```python
from build123d import *

# Parameters (mm, degrees)
BOSS_EXTRUDE1_DEPTH            = 3
SKETCH2_R                      = 3.5
BOSS_EXTRUDE2_DEPTH            = 1.5
M3_CLEARANCE_HOLE1_D           = 3.6
M3_CLEARANCE_HOLE1_ON_FACE_2_D = 3.6


with BuildPart() as part:
    # Sketch1 → Boss-Extrude1 (new body)
    with BuildSketch(Plane.XY):
        with BuildLine():
            Line((-15.5, 23), (15.5, 23))
            ThreePointArc((15.5, 23), (20.803300859, 20.803300859), (23, 15.5))
            Line((23, 15.5), (23, -15.5))
            ThreePointArc((23, -15.5), (20.803300859, -20.803300859), (15.5, -23))
            Line((15.5, -23), (-15.5, -23))
            ThreePointArc((-15.5, -23), (-20.803300859, -20.803300859), (-23, -15.5))
            Line((-23, -15.5), (-23, 15.5))
            ThreePointArc((-23, 15.5), (-20.803300859, 20.803300859), (-15.5, 23))
        make_face()
    extrude(amount=BOSS_EXTRUDE1_DEPTH)

    # Sketch2 → Boss-Extrude2 (add)
    with BuildSketch(Plane.XY.offset(3)):
        Circle(SKETCH2_R)
    extrude(amount=BOSS_EXTRUDE2_DEPTH)

    # M3 Clearance Hole1 (through all)
    with Locations(Plane(origin=(0, 0, 0), x_dir=(-1, 0, 0), z_dir=(0, 0, -1))):
        with Locations((0, 0)):
            Hole(M3_CLEARANCE_HOLE1_D / 2)

    # M3 Clearance Hole1 on face 2 (through all)
    with Locations(Plane.XY.offset(4.5)):
        with Locations((0, 0)):
            Hole(M3_CLEARANCE_HOLE1_ON_FACE_2_D / 2)


solid = part.part
```
Geometry check sheet. Reference: the model listing, model coordinates, mm. A direction names the side the tool comes from. Give positions to 0.01 mm unless a question says otherwise; leave off trailing zeros. Order: outer loops, then holes, each group sorted by start corner. A loop starts at its lowest first (then second) coordinate and runs counter-clockwise, first axis right, second up. Notation, with made-up numbers: (-5.5, 7.25) -> (1.5, 7.25) arc R27 cw to (1.5, 45.25) -> close; hole circle Ø4 at (67.5, 68). An arc over 180 degrees is marked (long way). Write each question's results on one line, items separated by ' | '. Start each with the question number.
(1) Mould release check, pull along Y, two halves, no side actions. Record for faces 1 (the face through (5, 0, 0)), 2 (the face through (-20.745, -20.861, 1.479)), 3 (the face through (1.717, 0.541, 2.281)): pulls with the +Y half, pulls with the -Y half, needs draft (parallel to the pull), parting line crosses it, or undercut.
(2) Sectioned sample at C-C (z = 3.7). Enter the section's corners in (x, y).
(3) Gauge pin test, flat ends, axial feed: P1, Ø23, axis at x = 6.5, y = 2.5, coming from the +Z side; P2, Ø1, axis at y = -17, z = 0.5, coming from the +X side; P3, Ø3, axis at x = 0, y = 0, coming from the -Z side; P4, Ø4, axis at x = -5.5, y = 5.5, coming from the +Z side. Record the tip position at first contact, or that the pin passes through.
(4) Sectioned sample at D-D (x = 8). Enter the section's corners in (y, z), plus the area to 3 significant figures.
(5) Scan lines: line 1 (Y direction, x = 0, z = 1.6); line 2 (Z direction, x = -4, y = 1.5); line 3 (X direction, y = -0.5, z = 0.65). Record each from-to range of solid material in increasing order.
(6) Access from +Z, -Z, +X, -X, +Y, -Y to the whole of each face (thin tool, end or side, straight path). Record for faces 4 (the face through (3.233, -1.341, 3.74)), 5 (the face through (23, 0, 1)).
(7) Sectioned sample at A-A (y = 0). Enter the section's corners in (x, z).
Answer below:
1) face 1: needs draft | face 2: pulls with the -Y half | face 3: undercut
2) outline: circle Ø7 at (0, 0); hole circle Ø3.6 at (0, 0)
3) P1: z = 4.5 | P2: x = 22.93 | P3: through | P4: z = 3
4) outline: (-23, 0) -> (23, 0) -> (23, 3) -> (-23, 3) -> close | area: 138 mm2
5) line 1: -23 to -1.8, 1.8 to 23 | line 2: 0 to 3 | line 3: -23 to -1.73, 1.73 to 23
6) face 4: +Z | face 5: +Z, -Z, +X, +Y, -Y
7) outline: (-23, 0) -> (-1.8, 0) -> (-1.8, 4.5) -> (-3.5, 4.5) -> (-3.5, 3) -> (-23, 3) -> close; (1.8, 0) -> (23, 0) -> (23, 3) -> (3.5, 3) -> (3.5, 4.5) -> (1.8, 4.5) -> close
